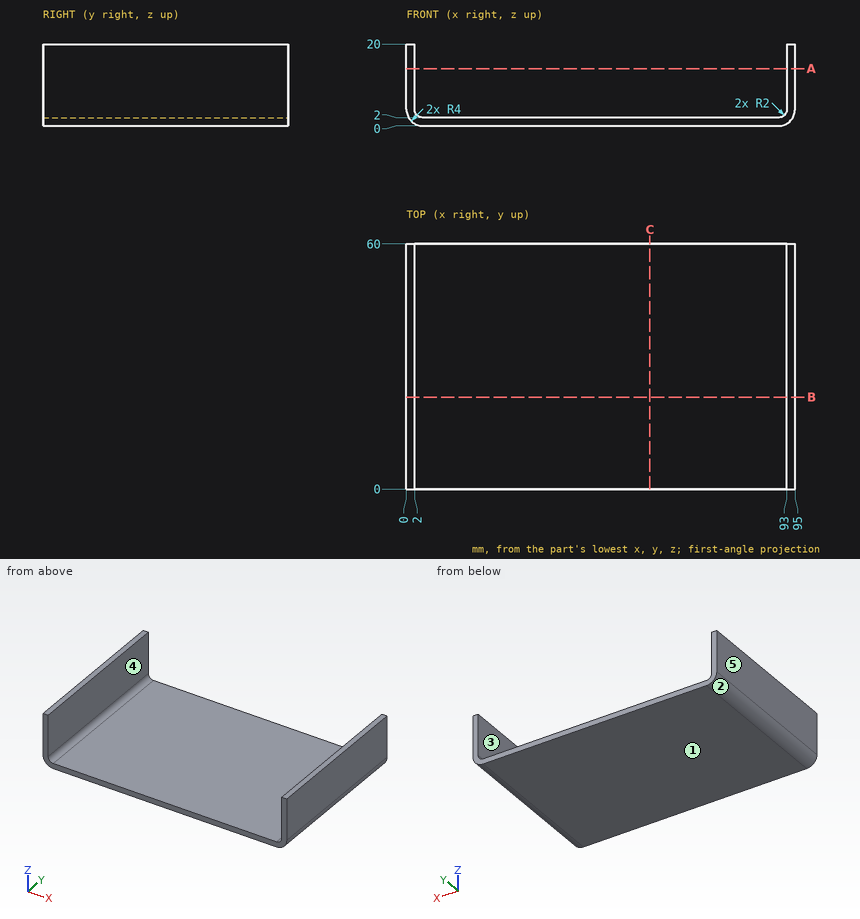
Design review of the part shown in the three views and the two pictorial views. Dimensions are in mm from the part's minimum x, y and z. A direction names the side the tool comes from. Round coordinates to 2 decimals unless told otherwise and drop trailing zeros. Loops run counter-clockwise (first coordinate to the right, second up) from the corner with the lowest first, then second, coordinate; pieces in that order, holes last.
(1) We need section B-B (y = 22.5). Give the boundary of the cut face in (x, z).
Returned:
outline: (0, 4) arc R4 ccw to (4, 0) - (91, 0) arc R4 ccw to (95, 4) - (95, 20) - (93, 20) - (93, 4) arc R2 cw to (91, 2) - (4, 2) arc R2 cw to (2, 4) - (2, 20) - (0, 20) - close
(2) Clearance check with a flat-ended pin moving along its axis: P1, Ø10, axis at x = 33, y = 20.5, coming from the +Z side. State where the tip first meets the part, or that it passes through.
Returned:
P1: stops at z = 2
(3) Wall thickness on line 1 along X through (y, z) = (9, 10); line 2 along Z through (x, y) = (31, 17): over which ranges is each line inside the solid? List them lowest first.
Returned:
line 1: x = 0 to 2, 93 to 95
line 2: z = 0 to 2
(4) We need section C-C (x = 59.5). Give the boundary of the cut face in (y, z), plus the area to 3 significant figures.
Returned:
outline: (0, 0) - (60, 0) - (60, 2) - (0, 2) - close
area: 120 mm2
(5) We need section A-A (z = 14). Give the boundary of the cut face in (x, y).
Returned:
outline: (0, 0) - (2, 0) - (2, 60) - (0, 60) - close; (93, 0) - (95, 0) - (95, 60) - (93, 60) - close
(6) Mouldability with a two-part tool opening along X and no side actions: class the marked faces 1, 2 and 3 as released by +X, released by -X, zero draft, split by the parting line, or undercut.
Returned:
face 1: zero draft
face 2: released by -X
face 3: undercut
(7) Tool access review of the marked faces 4 and 5: name each direction out of +Z, -Z, +X, -X, +Y, -Y from which nothing blocks a thin tool from reaching the whole face with its end or side.
Returned:
face 4: +Z, +Y, -Y
face 5: +Z, -Z, -X, +Y, -Y
